CAD build for the part. Positions are in the model's coordinates, mm. Face numbers are marked on the shaded views. A direction names the side the tool comes from. Round coordinates to 2 decimals unless told otherwise and drop trailing zeros. Loops run counter-clockwise (first coordinate to the right, second up) from the corner with the lowest first, then second, coordinate; pieces in that order, holes last.
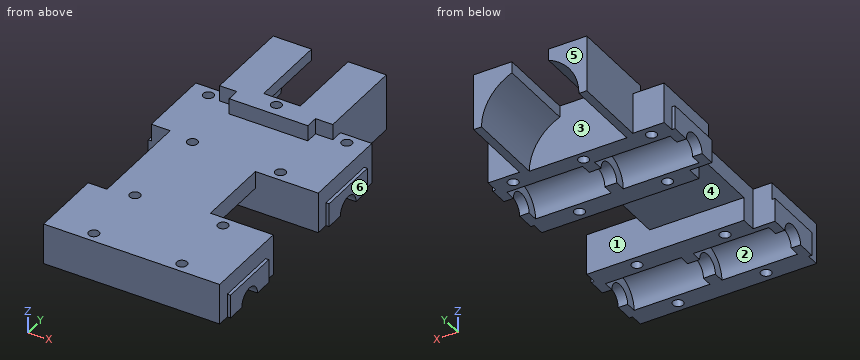
Autodesk Inventor part; units mm, degrees
ref_plane "작업 평면3" through (28, 11.75, -13) normal (0, 0, -1) x (-1, 0, 0)
ref_plane "YZ Plane" through (0, 0, 0) normal (1, 0, 0) x (0, 1, 0)
ref_plane "XZ Plane" through (0, 0, 0) normal (0, 1, 0) x (-1, 0, 0)
sketch "스케치1" plane through (0, 0, 0) normal (1, 0, 0) x (0, 1, 0)
  arc A0 (33.25, -13) -> (18.25, -13) centre (25.75, -13) ccw
  arc A1 (-18.25, -13) -> (-33.25, -13) centre (-25.75, -13) ccw
  line L0 (-37.5, 0) -> (35.75, 0)
  line L1 (33.25, -13) -> (35.75, -13)
  line L2 (18.25, -13) -> (15.75, -13)
  line L3 (15.75, -13) -> (15.75, -5.5)
  line L4 (-18.25, -13) -> (-15.75, -13)
  line L5 (-15.75, -13) -> (-15.75, -5.5)
  line L6 (-33.25, -13) -> (-35.75, -13)
  line L7 (-35.75, -13) -> (-35.75, -5.5)
  line L8 (-15.75, -13) -> (-11.75, -13)
  line L9 (-11.75, -13) -> (-11.75, -5.5)
  line L10 (-35.75, -13) -> (-39.75, -13)
  line L11 (-39.75, -13) -> (-39.75, -5.5)
  line L12 (15.75, -13) -> (11.75, -13)
  line L13 (11.75, -13) -> (11.75, -5.5)
  line L14 (35.75, -13) -> (39.75, -13)
  line L15 (25.75, -5.5) -> (15.75, -5.5)
  line L16 (35.75, -5.5) -> (25.75, -5.5)
  line L17 (15.75, -5.5) -> (11.75, -5.5)
  line L18 (11.75, -5.5) -> (-11.75, -5.5)
  line L19 (-15.75, -5.5) -> (-25.75, -5.5)
  line L20 (-35.75, -5.5) -> (-25.75, -5.5)
  line L21 (-11.75, -5.5) -> (-15.75, -5.5)
  arc A2 (29.85, -13) -> (21.65, -13) centre (25.75, -13) ccw
  line L22 (33.25, -13) -> (29.85, -13)
  line L23 (21.65, -13) -> (18.25, -13)
  arc A3 (-21.65, -13) -> (-29.85, -13) centre (-25.75, -13) ccw
  line L24 (-18.25, -13) -> (-21.65, -13)
  line L25 (-29.85, -13) -> (-33.25, -13)
  line L26 (29.85, -13) -> (21.65, -13)
  line L27 (-21.65, -13) -> (-29.85, -13)
  line L28 (35.75, 2) -> (60.75, 2)
  line L29 (60.75, 2) -> (60.75, -13)
  line L30 (35.75, 2) -> (35.75, 0)
  line L31 (35.75, 2) -> (35.75, 5)
  line L32 (35.75, 5) -> (60.75, 5)
  line L33 (60.75, 5) -> (63.75, 5)
  line L34 (63.75, 5) -> (63.75, 2)
  line L35 (63.75, 2) -> (63.75, -13)
  line L36 (63.75, -13) -> (60.75, -13)
  line L37 (-37.5, 0) -> (-39.75, 0)
  line L38 (-39.75, 0) -> (-39.75, -5.5)
  line L39 (-35.75, -5.5) -> (-35.75, 0)
  line L40 (39.75, 0) -> (39.75, -13)
  line L41 (35.75, 0) -> (35.75, -5.5)
  line L42 (35.75, -13) -> (35.75, -5.5)
  line L43 (39.75, 0) -> (39.75, 2)
  line L44 (60.75, -13) -> (39.75, -13)
  line L45 (35.75, 5) -> (31.75, 5)
  line L46 (31.75, 5) -> (31.75, 0)
  line L47 (39.75, 0) -> (35.75, 0)
  point P0 (0, 0)
  dimension "d1" = 37.5
  dimension "d8" = 2.5
  dimension "d10" = 2.5
  dimension "d11" = 4
  dimension "d12" = 4
  dimension "d13" = 4
  dimension "d28" = 8.2
  dimension "d29" = 8.2
  dimension "d37" = 25
  dimension "d38" = 3
  dimension "d39" = 3
  dimension "d81" = 4
extrude "돌출1" add sketch "스케치1" along normal mid plane 56 contours L15 L17 L18 L21 L19 L20 L39 L0 L41 L16
extrude "돌출3" add sketch "스케치1" along normal mid plane 56 contours L3 L12 L13 L17 | L9 L8 L5 L21
extrude "돌출4" add sketch "스케치1" along normal mid plane 56 contours L15 L17 L18 L21 L19 L20 L39 L0 L41 L16 | L39 L7 L10 L11 L38 L37 L0
extrude "돌출5" add sketch "스케치1" along normal mid plane 52 contours A0 L16 L42 L1 | A0 L2 L3 L15 | L5 L4 A1 L19 | A1 L6 L7 L20
extrude "돌출6" add sketch "스케치1" along normal mid plane 3.8 contours L22 A2 L23 A0 | A1 L24 A3 L25
sketch "스케치3" plane through (26, 0, 0) normal (1, 0, 0) x (0, 0, -1)
  line L0 (5.5, 15.75) -> (5.5, 35.75)
  line L1 (13, 11.75) -> (13, 15.75)
  line L2 (5.5, 35.75) -> (13, 35.75)
  line L3 (13, 15.75) -> (5.5, 15.75)
  line L4 (5.5, 15.75) -> (5.5, 35.75)
  line L5 (13, 18.25) -> (13, 21.65)
  arc A0 (13, 29.85) -> (13, 21.65) centre (13, 25.75) ccw
  line L6 (13, 35.75) -> (13, 29.85)
  line L7 (13, 21.65) -> (13, 15.75)
  line L8 (5.5, -15.75) -> (13, -15.75)
  line L9 (13, -35.75) -> (13, -39.75)
  line L10 (5.5, -15.75) -> (13, -15.75)
  line L11 (13, -35.75) -> (5.5, -35.75)
  line L12 (5.5, -35.75) -> (5.5, -15.75)
  line L13 (13, -33.25) -> (13, -29.85)
  arc A1 (13, -21.65) -> (13, -29.85) centre (13, -25.75) ccw
  line L14 (13, -15.75) -> (13, -21.65)
  line L15 (13, -29.85) -> (13, -35.75)
  point P0 (0, 0)
extrude "돌출8" add sketch "스케치3" along normal blind 3
sketch "스케치4" plane through (-26, 0, 0) normal (-1, 0, 0) x (0, 0, 1)
  line L0 (-13, -33.25) -> (-13, -35.75)
  line L1 (-5.5, -15.75) -> (-13, -15.75)
  line L2 (-13, -15.75) -> (-13, -35.75)
  line L3 (-13, -35.75) -> (-5.5, -35.75)
  line L4 (-5.5, -35.75) -> (-5.5, -15.75)
  line L5 (-13, 11.75) -> (-13, 15.75)
  line L6 (-5.5, 35.75) -> (0, 35.75)
  line L7 (-13, 15.75) -> (-5.5, 15.75)
  line L8 (-5.5, 15.75) -> (-5.5, 35.75)
  line L9 (-5.5, 35.75) -> (-13, 35.75)
  arc A0 (-13, -29.85) -> (-13, -21.65) centre (-13, -25.75) ccw
  arc A1 (-13, 21.65) -> (-13, 29.85) centre (-13, 25.75) ccw
  line L10 (-13, 35.75) -> (-13, 29.85)
  line L11 (-13, 21.65) -> (-13, 15.75)
  point P0 (0, 0)
extrude "돌출9" add sketch "스케치4" along normal blind 3 contours L2 A0 L1 L4 L3 L0 | L11 A1 L10 L9 L8 L7
extrude "돌출10" add sketch "스케치1" along normal mid plane 36 contours A0 L16 L42 L1 | L29 L28 L31 L32 L33 L34 L35 L36
sketch "스케치5" plane through (-18, 63.75, 5) normal (0, 1, 0) x (1, 0, 0)
  line L0 (0, 18) -> (36, 18)
  arc A0 (2.5, 18) -> (33.5, 18) centre (18, 18) ccw
  line L1 (18, 18) -> (2.5, 18)
  line L2 (-10, 18) -> (46, 18)
  line L3 (18, 18) -> (33.5, 18)
  line L4 (-10, 5) -> (46, 5)
  line L5 (23.8125, 3.6311) -> (23.8125, 0)
  line L6 (23.8125, 3.6311) -> (12.1875, 3.6311)
  line L7 (12.1875, 0) -> (23.8125, 0)
  line L8 (12.1875, 3.6311) -> (12.1875, 0)
  point P0 (18, 5)
  dimension "d43" = 31
sketch "스케치6" plane through (28, 11.75, -13) normal (0, 0, -1) x (-1, 0, 0)
  line L0 (28, 0) -> (28, 3.25)
  line L1 (28, 3.25) -> (14, 3.25)
  line L2 (28, 3.25) -> (42, 3.25)
  circle A0 centre (42, 3.25) radius 1.65
  circle A1 centre (14, 3.25) radius 1.65
  line L3 (28, 24.75) -> (6, 24.75)
  line L4 (28, 24.75) -> (50, 24.75)
  circle A2 centre (6, 24.75) radius 1.65
  circle A3 centre (50, 24.75) radius 1.65
  line L5 (28, 21.5) -> (28, 24.1)
  circle A4 centre (28, 24.1) radius 1.65
  line L6 (0, -23.5) -> (56, -23.5)
  line L7 (28, -23.5) -> (28, -26.75)
  line L8 (28, -26.75) -> (42, -26.75)
  line L9 (28, -26.75) -> (14, -26.75)
  line L10 (56, -51.5) -> (0, -51.5)
  line L11 (28, -51.5) -> (28, -48.25)
  line L12 (28, -48.25) -> (42, -48.25)
  line L13 (28, -48.25) -> (14, -48.25)
  circle A5 centre (14, -26.75) radius 1.65
  circle A6 centre (42, -26.75) radius 1.65
  circle A7 centre (42, -48.25) radius 1.65
  circle A8 centre (14, -48.25) radius 1.65
  point P0 (28, -11.75)
  dimension "d46" = 3.25
  dimension "d47" = 14
  dimension "d48" = 14
  dimension "d54" = 3.3
  dimension "d55" = 3.3
  dimension "d58" = 22
  dimension "d59" = 3.3
  dimension "d60" = 3.3
  dimension "d61" = 2.6
  dimension "d62" = 3.3
  dimension "d63" = 3.25
  dimension "d64" = 14
  dimension "d65" = 14
  dimension "d66" = 3.25
  dimension "d67" = 14
  dimension "d68" = 14
  dimension "d69" = 3.3
  dimension "d70" = 3.3
  dimension "d71" = 3.3
  dimension "d72" = 3.3
extrude "돌출13" add sketch "스케치1" along normal mid plane 56 contours L42 L41 L47 L40 L14 | L30 L28 L43 L47
extrude "돌출14" add sketch "스케치1" along normal mid plane 36 contours L40 L43 L28 L29 L44
extrude "돌출15" cut sketch "스케치5" against normal blind 25 contours L0 A0 L4 | L4 A0 L6 | L6 A0
extrude "돌출16" add sketch "스케치1" along normal mid plane 25 contours L0 L46 L45 L31 L30
extrude "돌출17" cut sketch "스케치6" against normal blind 20
sketch "스케치7" plane through (-28, 39.75, 2) normal (0, 0, 1) x (1, 0, 0)
  line L0 (0, -79.5) -> (0, -4)
  line L1 (0, 0) -> (10, 0)
  line L2 (0, -4) -> (10, -4)
  line L3 (10, -4) -> (10, 0)
  line L4 (10, 0) -> (0, 0)
  line L5 (0, 0) -> (0, -4)
  line L6 (46, -4) -> (46, 0)
  line L7 (46, -4) -> (56, -4)
  line L8 (56, -4) -> (56, 0)
  line L9 (56, 0) -> (46, 0)
  line L10 (46, 0) -> (46, -4)
  point P0 (28, -39.75)
extrude "돌출18" cut sketch "스케치7" against normal blind 2
sketch "스케치8" plane through (28, 11.75, -5.5) normal (0, 0, -1) x (-1, 0, 0)
  line L0 (0, -23.5) -> (56, -23.5)
  line L1 (46, -23.5) -> (41, -23.5)
  line L2 (56, -23.5) -> (0, -23.5)
  line L3 (0, -23.5) -> (6, -23.5)
  line L4 (6, -23.5) -> (6, 0)
  line L5 (0, -23.5) -> (0, 0)
  line L6 (0, 0) -> (0, -23.5)
  line L7 (0, 0) -> (6, 0)
  line L8 (6, -1.75) -> (0, -1.75)
  line L9 (6, -8.25) -> (0, -8.25)
  line L10 (6, -15.25) -> (0, -15.25)
  line L11 (6, -21.75) -> (0, -21.75)
  line L12 (57, -11.75) -> (50, -11.75)
  line L13 (50, -11.75) -> (50, 4.75)
  line L14 (50, 4.75) -> (57, 4.75)
  line L15 (50, 4.75) -> (57, 4.75)
  line L16 (57, -11.75) -> (57, 4.75)
  line L17 (50, -11.75) -> (50, -28.25)
  line L18 (50, -28.25) -> (57, -28.25)
  line L19 (57, -11.75) -> (57, -28.25)
  line L20 (56, 0) -> (56, -23.5)
  point P0 (28, -11.75)
  dimension "d115" = 6
  dimension "d147" = 7
  dimension "d148" = 16.5
  dimension "d149" = 16.5
ref_plane "작업 평면3" through (28, 11.75, -13) normal (0, 0, -1) x (-1, 0, 0)
extrude "돌출28" cut sketch "스케치5" against normal blind 25 contours A0 L5 L7 L8
extrude "돌출29" cut sketch "스케치8" along normal mid plane 20 contours L17 L12 L20 L0 | L0 L20 L12 L19 L18 L17 | L13 L14 L16 L12
sketch "스케치15" plane through (28, -11.75, -5.5) normal (0, 0, -1) x (-1, 0, 0)
  line L0 (0, -4) -> (0, 0)
  line L1 (50, 23.5) -> (0, 23.5)
  line L2 (0, 0) -> (20, 0)
  line L3 (20, 0) -> (20, 23.5)
  line L4 (20, 23.5) -> (0, 23.5)
  line L5 (0, 23.5) -> (0, 0)
  point P0 (28, 11.75)
  dimension "d152" = 20
extrude "돌출30" cut sketch "스케치15" against normal blind 10
properties part number "x 캐리지"
Item 1: Flat gauge pins, fed straight in: P1, Ø8, axis at y = 23, z = 2.5, coming from the -X side; P2, Ø4, axis at y = -8.5, z = -3.5, coming from the +X side; P3, Ø2.5, axis at x = 15, z = 2.5, coming from the -Y side. Where does each tip first touch, or does it go through?
Verdict:
P1: stops at x = -28
P2: stops at x = 8
P3: stops at y = 35.75
Item 2: Cut at D-D (z = -10). State how many separate pieces and enclosed holes the cut face has, plus the area to 3 significant figures.
Verdict:
separate pieces: 4
enclosed holes: 9
area: 1,750 mm2
Item 3: 3-axis set-ups, long thin cutter, end or side, ignore diameter. For the marked faces 1, 2 and 3: which of +Z, -Z, +X, -X, +Y, -Y reach the whole face in a straight line?
Verdict:
face 1: -Z, +X
face 2: -Z
face 3: -Z, +Y
Item 4: Cut at B-B (x = 9). List the corners of the cut face in (y, z).
Verdict:
outline: (-39.75, -13) - (-33.25, -13) arc R7.5 cw to (-18.25, -13) - (-11.75, -13) - (-11.75, 0) - (-39.75, 0) - close; (11.75, -13) - (18.25, -13) arc R7.5 cw to (33.25, -13) - (38.75, -13) - (38.75, -0.38) - (63.75, -0.38) - (63.75, 5) - (31.75, 5) - (31.75, 0) - (11.75, 0) - close
Item 5: Cut at C-C (y = 51). List the corners of the cut face in (x, z).
Verdict:
outline: (-18, -13) - (-15.5, -13) arc R15.5 cw to (-5.81, 1.37) - (-5.81, 5) - (-18, 5) - close; (5.81, 1.37) arc R15.5 cw to (15.5, -13) - (18, -13) - (18, 5) - (5.81, 5) - close
Item 6: Mould opens along Y. For the marked faces 4, 5 and 6 say: released by +Y, released by -Y, zero draft, split by the parting line, or undercut.
Verdict:
face 4: undercut
face 5: released by +Y
face 6: zero draft
Item 7: Cut at A-A (y = -25.75). List the corners of the cut face in (x, z).
Verdict:
outline: (-29, -8.9) - (-26, -8.9) - (-26, -5.5) - (-1.9, -5.5) - (-1.9, -8.9) - (1.9, -8.9) - (1.9, -5.5) - (26, -5.5) - (26, -8.9) - (29, -8.9) - (29, -5.5) - (28, -5.5) - (28, 0) - (-28, 0) - (-28, -5.5) - (-29, -5.5) - close
Item 8: Wall check: L1, parallel to Y at x = -14, z = -4.75; L2, parallel to Y at x = 14, z = -4.75; L3, parallel to X at y = 35.85, z = -4. Give the ranges that are in metal, low to high.
Verdict:
L1: y = -39.75 to -38.15, -34.85 to -16.65, -13.35 to 13.35, 16.65 to 63.75
L2: y = -39.75 to -38.15, -34.85 to -16.65, -13.35 to -11.75, 11.75 to 13.35, 16.65 to 63.75
L3: x = -28 to -23.52, -20.48 to -1.65, 1.65 to 20.48, 23.52 to 28
